The figure shows three views and two pictorial views of one solid part (mm, origin at its lowest corner). Answer the questions. A direction names the side the tool comes from. Round coordinates to 2 decimals unless told otherwise and drop trailing zeros. Write each loop counter-clockwise with the first axis right and the second up, starting at its lowest first coordinate (ties: lowest second). Pieces come first, ordered by that corner, then holes. Notation, with made-up numbers: (31.5, 35) -> (56.5, 35) arc R31 ccw to (56.5, 68) -> close; hole circle Ø5 at (84.5, 9). An arc over 180 degrees is marked (long way). One line per item, written item: value.
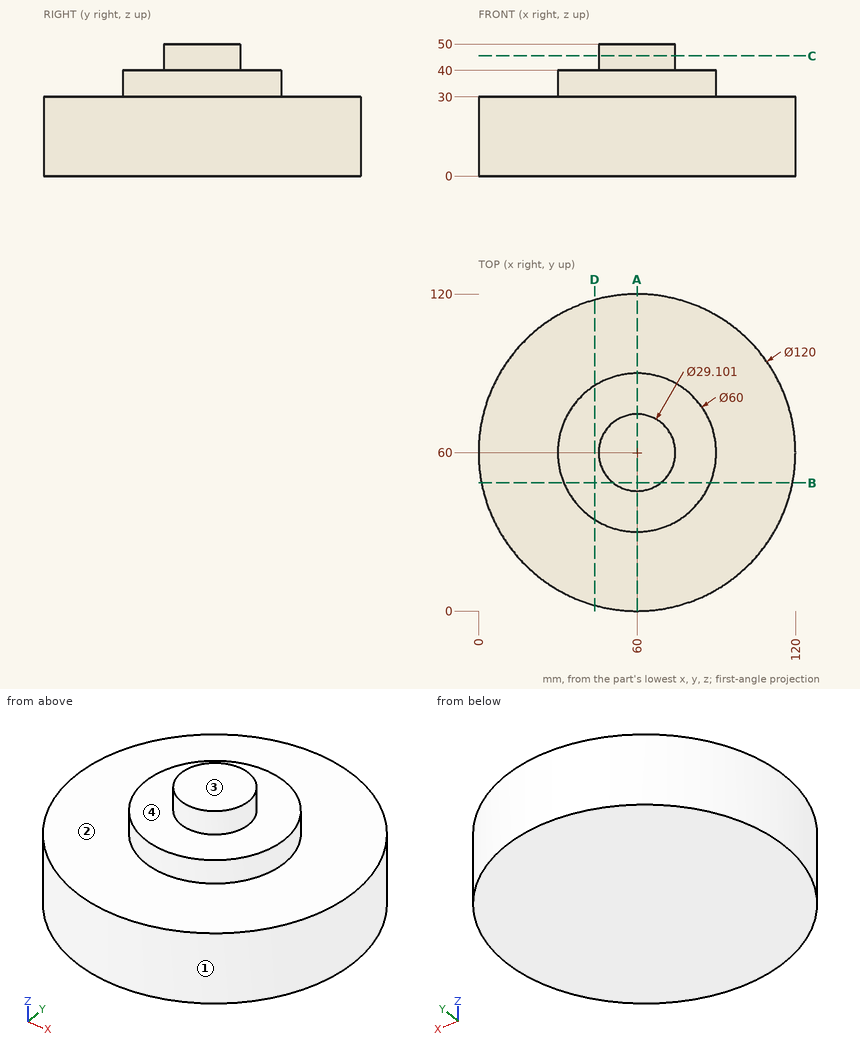
(1) Find section B-B on y = 48.5. Give the vertices of the cut face in (x, z), plus the area to 3 significant figures.
Reported:
outline: (1.11, 0) -> (118.89, 0) -> (118.89, 30) -> (87.71, 30) -> (87.71, 40) -> (68.91, 40) -> (68.91, 50) -> (51.09, 50) -> (51.09, 40) -> (32.29, 40) -> (32.29, 30) -> (1.11, 30) -> close
area: 4,270 mm2
(2) Find section C-C on z = 45.5. Give the vertices of the cut face in (x, y).
Reported:
outline: circle Ø29.1 at (60, 60)
(3) A tool of negligible diameter and unlimited length cuts with its end or side. For the marked faces 3 and 4, from which of +Z, -Z, +X, -X, +Y, -Y can it reach the whole face along a straight path? Write none if from no direction.
Reported:
face 3: +Z, +X, -X, +Y, -Y
face 4: +Z
(4) Find section A-A on x = 60. Give the vertices of the cut face in (y, z).
Reported:
outline: (0, 0) -> (120, 0) -> (120, 30) -> (90, 30) -> (90, 40) -> (74.55, 40) -> (74.55, 50) -> (45.45, 50) -> (45.45, 40) -> (30, 40) -> (30, 30) -> (0, 30) -> close
(5) For a pull along Y with two mould halves and no side action, classify the marked faces 1 and 2 as pulls with the +Y half, pulls with the -Y half, needs draft (parallel to the pull), parting line crosses it, or undercut.
Reported:
face 1: parting line crosses it
face 2: needs draft
(6) Find section D-D on x = 44. Give the vertices of the cut face in (y, z).
Reported:
outline: (2.17, 0) -> (117.83, 0) -> (117.83, 30) -> (85.38, 30) -> (85.38, 40) -> (34.62, 40) -> (34.62, 30) -> (2.17, 30) -> close
(7) Consider probe 1 along Z at (x, y) = (21.5, 100); probe 2 along Z at (x, y) = (43, 61.5); probe 3 along X at (y, z) = (52.5, 27). Determine where each line is inside the solid, lowest interval first.
Reported:
probe 1: z = 0 to 30
probe 2: z = 0 to 40
probe 3: x = 0.47 to 119.53
(8) Flat-ended cylindrical pins translate along their axes: pin 1 Ø2 at (y, z) = (23.5, 19) entering from +X; pin 2 Ø1.5 at (x, z) = (79.5, 21.5) entering from -Y; pin 3 Ø3 at (x, z) = (73, 34.5) entering from +Y. Find the tip coordinate at first contact, or state that the pin passes through.
Reported:
pin 1: stops at x = 108.37
pin 2: stops at y = 3
pin 3: stops at y = 87.71
